```python
from build123d import *

# Parameters (mm, degrees)
F1_DEPTH = 6
F2_SIZE  = 0.5
F3_SIZE  = 0.3
F4_R     = 3.555
F5_DEPTH = 2.5
F6_R     = 2.5
F7_DEPTH = 8.501


with BuildPart() as f1:
    # F0 (on Top) → F1 (new body)
    with BuildSketch(Plane.XY):
        Polygon((0, -5.7735026919), (5, -2.8867513459), (5, 2.8867513459), (0, 5.7735026919), (-5, 2.8867513459), (-5, -2.8867513459), align=None)
    extrude(amount=F1_DEPTH)

    # F2
    f2_edges = [f1.edges().sort_by_distance(p)[0] for p in [
        (5, 2.886751, 3),
        (0, 5.773503, 3),
        (5, -2.886751, 3),
        (0, -5.773503, 3),
        (-5, -2.886751, 3),
        (-5, 2.886751, 3),
    ]]
    chamfer(f2_edges, length=F2_SIZE)

    # F3
    f3_edges = [f1.edges().sort_by_distance(p)[0] for p in [
        (4.783494, 2.761751, 6),
        (4.783494, -2.761751, 6),
        (0, 5.523503, 6),
        (-4.783494, 2.761751, 6),
        (-4.783494, -2.761751, 6),
        (0, -5.523503, 6),
        (-4.783494, -2.761751, 0),
        (0, -5.523503, 0),
        (4.783494, -2.761751, 0),
        (4.783494, 2.761751, 0),
        (0, 5.523503, 0),
        (-4.783494, 2.761751, 0),
    ]]
    chamfer(f3_edges, length=F3_SIZE)

    # F4 (on face) → F5 (join)
    with BuildSketch(Plane.XY.offset(6)):
        Circle(F4_R)
    extrude(amount=F5_DEPTH)

    # F6 (on face) → F7 (cut, through all)
    with BuildSketch(Plane.XY.offset(8.5)):
        with Locations((0.79, 0)):
            Circle(F6_R)
    extrude(amount=-F7_DEPTH, mode=Mode.SUBTRACT)


solid = f1.part
```
CAD build for the part. Positions are in the model's coordinates, mm. A direction names the side the tool comes from. Give positions to 0.01 mm unless a question says otherwise; leave off trailing zeros. Loops run counter-clockwise (first coordinate to the right, second up) from the corner with the lowest first, then second, coordinate; pieces in that order, holes last. Notation, with made-up numbers: M -16.75,47 L 6.25,47 A25 ccw 6.25,77 Z; hole C 38.5,71.25 d2. An arc over 180 degrees is marked long. Use one line per item in the form item = value.
Item 1: Which spindle directions (+Z, -Z, +X, -X, +Y, -Y) get a long thin tool onto all of the face, cutting with end or side? Do faces 1 (the face through (2.529, 4.313, 2.958)), 2 (the face through (0, 4, 6)). Say none if no direction does.
Determined:
face_1 = +Z, -Z, +X, +Y
face_2 = +Z
Item 2: Flat gauge pin, fed straight in: pin 1 (5 mm diameter, centred on x = -3, z = 4.5, fed in from +Y). Where does the tip first touch, or does it go through?
Determined:
pin_1 = 5.48
Item 3: Slice it at C-C (x = -0.75). List the corners of the cut face in (y, z), plus the area to 3 significant figures.
Determined:
outline = M -5.34,0.12 L -5.22,0 L -1.97,0 L -1.97,8.5 L -3.47,8.5 L -3.47,6 L -5.22,6 L -5.34,5.88 Z; M 1.97,0 L 5.22,0 L 5.34,0.12 L 5.34,5.88 L 5.22,6 L 3.47,6 L 3.47,8.5 L 1.97,8.5 Z
area = 48.0 mm2
Item 4: Slice it at A-A (y = 0). List the corners of the cut face in (x, z) (3 decimals), plus the area to 3 significant figures.
Determined:
outline = M -5,0 L -1.71,0 L -1.71,8.5 L -3.555,8.5 L -3.555,6 L -5,6 Z; M 3.29,0 L 5,0 L 5,6 L 3.555,6 L 3.555,8.5 L 3.29,8.5 Z
area = 35.3 mm2
Item 5: Drill centre lines: probe 1 along X at (y, z) = (0.5, 3); probe 2 along Z at (x, y) = (3, -3.5); probe 3 along Y at (x, z) = (2, 0.5). Where is each one in solid material? Low to high. Write a range as from..to.
Determined:
probe_1 = -5..-1.66, 3.24..5
probe_2 = 0..6
probe_3 = -4.62..-2.19, 2.19..4.62
Item 6: Slice it at D-D (x = 0.79). List the corners of the cut face in (y, z), plus the area to 3 significant figures.
Determined:
outline = M -5.32,0.09 L -5.22,0 L -2.5,0 L -2.5,8.5 L -3.47,8.5 L -3.47,6 L -5.22,6 L -5.32,5.91 Z; M 2.5,0 L 5.22,0 L 5.32,0.09 L 5.32,5.91 L 5.22,6 L 3.47,6 L 3.47,8.5 L 2.5,8.5 Z
area = 38.6 mm2
Item 7: Slice it at B-B (z = 3). List the corners of the cut face in (x, y).
Determined:
outline = M -5,-2.39 L -4.57,-3.14 L -0.43,-5.52 L 0.43,-5.52 L 4.57,-3.14 L 5,-2.39 L 5,2.39 L 4.57,3.14 L 0.43,5.52 L -0.43,5.52 L -4.57,3.14 L -5,2.39 Z; hole C 0.79,0 d5
Item 8: Two-plate mould, pull along Y, no slides. Class faces 3 (the face through (-5, 0, 3)), 4 (the face through (-4.62, 2.68, 0.12)), 5 (the face through (0.25, -2.44, 4.31)): pulls with the +Y half, pulls with the -Y half, needs draft (parallel to the pull), parting line crosses it, or undercut.
Determined:
face_3 = needs draft
face_4 = pulls with the +Y half
face_5 = undercut
